The listing builds one solid part. Answer for the finished solid, in the listing's coordinates (mm). Face numbers are marked on the shaded views. A direction names the side the tool comes from. Round coordinates to 2 decimals unless told otherwise and drop trailing zeros. Write each loop counter-clockwise with the first axis right and the second up, starting at its lowest first coordinate (ties: lowest second). Pieces come first, ordered by that corner, then holes. Notation, with made-up numbers: (44, 65) - (72, 65) arc R4 cw to (72, 71) - close; hole circle Ø10 at (82.25, 68.5). An arc over 180 degrees is marked (long way). Use a Markdown table: item, result. Add a question column.
1) A tool of negligible diameter and unlimited length cuts with its end or side. For the marked faces 1, 2 and 3, from which of +Z, -Z, +X, -X, +Y, -Y can it reach the whole face along a straight path? Write none if from no direction.
2) Find the intervals of material crossed by probe 1 along Y at (x, z) = (33, -5.25); probe 2 along Z at (x, y) = (8.5, -2.5); probe 3 along Z at (x, y) = (72.5, 18), in increasing order. Write a range as from..to.
3) A cutting plane is placed at B-B (y = 3). Give the vertices of the cut face in (x, z).
4) A cutting plane is placed at A-A (y = 8). Give the vertices of the cut face in (x, z), then the cut area to 3 significant figures.
5) A cutting plane is placed at C-C (x = 11.5). Give the vertices of the cut face in (y, z), then the cut area to 4 significant figures.
6) Determine the mould class of the marked faces 4, 5, 6 and 7 for opening direction X: +X half, -X half, draft (parallel to the pull), parting line (faces both ways), or undercut.
7) Each of these flat-tipped pins is pushed along its axis until it touches: P1, Ø8, axis at y = 7.5, z = 52, coming from the +X side; P2, Ø2.5, axis at y = 8, z = -5.5, coming from the +X side; P3, Ø8, axis at x = 32.5, z = 46, coming from the -Y side; P4, Ø10, axis at x = 0, y = 0, coming from the +Z side. Where does it stop, or does it pass through?
8) A cutting plane is placed at D-D (y = -2). Give the vertices of the cut face in (x, z).
```python
from build123d import *

# Parameters (mm, degrees)
F0_R     = 5.5
F1_DEPTH = 9
F3_DEPTH = 9
F4_R     = 7
F5_DEPTH = 9


with BuildPart() as f1:
    # F0 (on Top) → F1 (new body)
    with BuildSketch(Plane.XY):
        with BuildLine():
            Line((46, 24), (-13, 24))
            Line((-13, 24), (-13, 0))
            ThreePointArc((-13, 0), (-9.1923881554, -9.1923881554), (0, -13))
            Line((0, -13), (33, -13))
            ThreePointArc((33, -13), (42.1923881554, -9.1923881554), (46, 0))
            Line((46, 0), (46, 24))
        make_face()
        Circle(F0_R, mode=Mode.SUBTRACT)
        with Locations((33, 0)):
            Circle(F0_R, mode=Mode.SUBTRACT)
    extrude(amount=-F1_DEPTH)

    # F2 (on face) → F3 (join)
    with BuildSketch(Plane(origin=(0, 24, 0), x_dir=(-1, 0, 0), z_dir=(0, 1, 0))):
        Polygon((-75.941125497, 43.686291501), (-46, -9), (-46, 0), (13, 0), (-53.313708499, 66.313708499), align=None)
    extrude(amount=-F3_DEPTH)

    # F4 (on face) → F5 (join)
    with BuildSketch(Plane(origin=(59.813708499, 0, 59.813708499), x_dir=(0.7071067812, 0, -0.7071067812), z_dir=(0.7071067812, 0, 0.7071067812))):
        with BuildLine():
            Line((22.8076118446, -5), (22.8076118446, 15))
            Line((22.8076118446, 15), (-9.1923881554, 15))
            Line((-9.1923881554, 15), (-9.1923881554, -5))
            ThreePointArc((-9.1923881554, -5), (6.8076118446, -21), (22.8076118446, -5))
        make_face()
        with Locations((6.8076118446, -5)):
            Circle(F4_R, mode=Mode.SUBTRACT)
    extrude(amount=-F5_DEPTH)


solid = f1.part
```
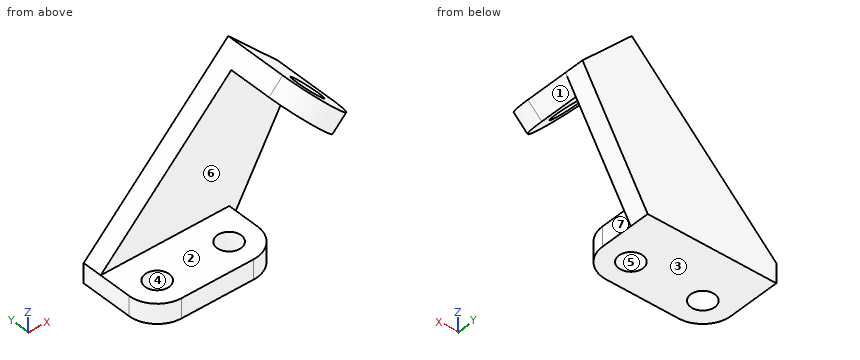
Entries:
| question | item | result |
|---|---|---|
| 1 | face 1 | -Z, +X, -Y |
| 1 | face 2 | +Z, +X, -X, -Y |
| 1 | face 3 | -Z, +X, -X, +Y, -Y |
| 2 | probe 1 | y = -13..-5.5, 5.5..24 |
| 2 | probe 2 | z = -9..0 |
| 2 | probe 3 | z = 37.63..47.13 |
| 3 | outline | (-13, -9) - (-4.61, -9) - (-4.61, 0) - (-13, 0) - close; (4.61, -9) - (28.39, -9) - (28.39, 0) - (4.61, 0) - close; (37.61, -9) - (46, -9) - (46, 0) - (37.61, 0) - close; (46.95, 59.95) - (69.58, 37.32) - (75.94, 43.69) - (53.31, 66.31) - close |
| 4 | outline | (-13, -9) - (46, -9) - (46, 0) - (-13, 0) - close; (46.95, 59.95) - (69.58, 37.32) - (75.94, 43.69) - (53.31, 66.31) - close |
| 4 | area | 819 mm² |
| 5 | outline | (-13, -9) - (24, -9) - (24, 24.5) - (15, 24.5) - (15, 0) - (-13, 0) - close |
| 5 | area | 553.5 mm² |
| 6 | face 4 | undercut |
| 6 | face 5 | undercut |
| 6 | face 6 | draft |
| 6 | face 7 | +X half |
| 7 | P1 | stops at x = 71.63 |
| 7 | P2 | stops at x = 46 |
| 7 | P3 | stops at y = 15 |
| 7 | P4 | passes through |
| 8 | outline | (-12.85, -9) - (-5.12, -9) - (-5.12, 0) - (-12.85, 0) - close; (5.12, -9) - (27.88, -9) - (27.88, 0) - (5.12, 0) - close; (38.12, -9) - (45.85, -9) - (45.85, 0) - (38.12, 0) - close; (46.95, 59.95) - (53.79, 53.11) - (60.16, 59.47) - (53.31, 66.31) - close; (62.74, 44.16) - (69.58, 37.32) - (75.94, 43.69) - (69.1, 50.53) - close |
